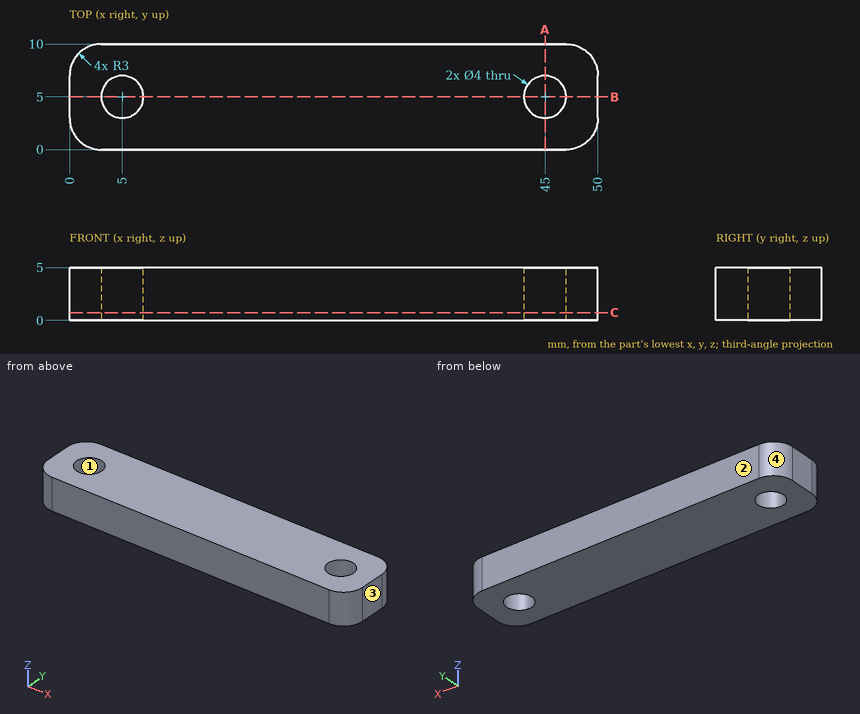
Print and shaded views of the part. All mm, measured from the part's lowest x, y and z. Coordinates: 2 decimals unless noted, no trailing zeros. Order: outer loops, then holes, each group sorted by start corner. A loop starts at its lowest first (then second) coordinate and runs counter-clockwise, first axis right, second up. Notation, with made-up numbers: (-26, 6) -> (28, 6) arc R18 cw to (28, 15) -> close; hole circle Ø7 at (-9, 89). An arc over 180 degrees is marked (long way). Answer as a JSON object with one key per item and string values. Group by question number.
1) Cut at A-A, the plane x = 45. Write the cut outline in (y, z).
2) Cut at B-B, the plane y = 5. Write the cut outline in (x, z), then the cut area to 3 significant figures.
3) Drill centre lines: L1, parallel to Y at x = 45, z = 2.7; L2, parallel to X at y = 4, z = 1.05; L3, parallel to X at y = 1.75, z = 1.8. Where is each one in solid material? Low to high.
4) Pull direction X, two halves, no side cores. Call the marked faces 1, 2, 3 and 4: +X half, -X half, draft (parallel to the pull), parting line (faces both ways), or undercut.
5) Cut at C-C, the plane z = 0.75. Write the cut outline in (x, y), then the cut area to 3 significant figures.
Check values:
{
 "1": {"outline": "(0, 0) -> (3, 0) -> (3, 5) -> (0, 5) -> close; (7, 0) -> (10, 0) -> (10, 5) -> (7, 5) -> close"},
 "2": {"outline": "(0, 0) -> (3, 0) -> (3, 5) -> (0, 5) -> close; (7, 0) -> (43, 0) -> (43, 5) -> (7, 5) -> close; (47, 0) -> (50, 0) -> (50, 5) -> (47, 5) -> close", "area": "210 mm²"},
 "3": {"L1": "y = 0 to 3, 7 to 10", "L2": "x = 0 to 3.27, 6.73 to 43.27, 46.73 to 50", "L3": "x = 0.27 to 49.73"},
 "4": {"face 1": "undercut", "face 2": "draft", "face 3": "+X half", "face 4": "-X half"},
 "5": {"outline": "(0, 3) arc R3 ccw to (3, 0) -> (47, 0) arc R3 ccw to (50, 3) -> (50, 7) arc R3 ccw to (47, 10) -> (3, 10) arc R3 ccw to (0, 7) -> close; hole circle Ø4 at (5, 5); hole circle Ø4 at (45, 5)", "area": "467 mm²"}
}
